from build123d import *

# Parameters (mm, degrees)
SKETCH_R     = 2.8
PAD_DEPTH    = 3
SKETCH001_R  = 1.45
PAD001_DEPTH = 16
POCKET_DEPTH = 2
CHAMFER_SIZE = 0.25


with BuildPart() as part:
    # Sketch → Pad (new body)
    with BuildSketch(Plane.XY):
        Circle(SKETCH_R)
    extrude(amount=PAD_DEPTH)

    # Sketch001 (on Face3 of Pad) → Pad001 (join)
    with BuildSketch(Plane.XY.offset(3)):
        Circle(SKETCH001_R)
    extrude(amount=PAD001_DEPTH)

    # Sketch002 (on Face2 of Pad001) → Pocket (cut)
    with BuildSketch(Plane(origin=(0, 0, 0), x_dir=(1, 0, 0), z_dir=(0, 0, -1))):
        Polygon((1.259542, 0.814588), (-0.075682, 1.49809), (-1.335225, 0.683502), (-1.259542, -0.814588), (0.075682, -1.49809), (1.335225, -0.683502), align=None)
    extrude(amount=-POCKET_DEPTH, mode=Mode.SUBTRACT)

    # Chamfer
    chamfer_edges = [part.edges().sort_by_distance(p)[0] for p in [
        (-2.8, 0, 3),
        (-2.8, 0, 0),
        (1.297384, -0.065543, 0),
        (0.705454, 1.090796, 0),
        (-0.59193, 1.156339, 0),
        (-1.297384, 0.065543, 0),
        (-0.705454, -1.090796, 0),
        (0.59193, -1.156339, 0),
        (-1.45, 0, 19),
    ]]
    chamfer(chamfer_edges, length=CHAMFER_SIZE)


solid = part.part
Read the model definition and answer for the solid it produces. Units are mm, in the model's axes. A direction names the side the tool comes from. Coordinates: 2 decimals unless noted, no trailing zeros. Loops run counter-clockwise (first coordinate to the right, second up) from the corner with the lowest first, then second, coordinate; pieces in that order, holes last.
Q1. Which of the six approach directions +Z, -Z, +X, -X, +Y, -Y give full straight-line access (tool end or side, diameter ignored) to faces 1 (the face through (0, 0, 19)), 2 (the face through (0, -2, 3)), 3 (the face through (0.697, 1.096, 1.113))?
Q2. The part is cut by section C-C on z = 2.25. Write down the section's boundary in (x, y).
Q3. The part is cut by section B-B on z = 6.25. Write down the section's boundary in (x, y).
Q4. Each of these flat-tipped pins is pushed along its axis until it touches: pin 1 Ø1 at (x, y) = (1.5, -1.5) entering from +Z; pin 2 Ø2 at (y, z) = (-0.5, 10.5) entering from +X; pin 3 Ø1 at (x, z) = (0.5, 8.5) entering from +Y. Where does it stop, or does it pass through?
Q5. The part is cut by section A-A on y = 0. Write down the section's boundary in (x, z), and give its area (3 significant figures).
Q6. The mould has two halves that part along X. Classify faces 4 (the face through (2, 0, 0)), 5 (the face through (-1.45, 0.06, 10.76)), 6 (the face through (-0.76, -1.2, 0.13)): +X half, -X half, draft (parallel to the pull), parting line (faces both ways), or undercut.
Q7. Consider probe 1 along Z at (x, y) = (1.6, -0.1); probe 2 along Y at (x, z) = (0.95, 4.25); probe 3 along Z at (x, y) = (-0.15, -1.15). Determine where each line is inside the solid, lowest interval first.
Results below:
1. face 1: +Z, +X, -X, +Y, -Y
1. face 2: +Z
1. face 3: -Z
2. outline: circle Ø5.6 at (0, 0)
3. outline: circle Ø2.9 at (0, 0)
4. pin 1: stops at z = 3
4. pin 2: stops at x = 1.45
4. pin 3: stops at y = 1.45
5. outline: (-2.8, 0.25) - (-2.55, 0) - (-1.55, 0) - (-1.3, 0.25) - (-1.3, 2) - (1.3, 2) - (1.3, 0.25) - (1.55, 0) - (2.55, 0) - (2.8, 0.25) - (2.8, 2.75) - (2.55, 3) - (1.45, 3) - (1.45, 18.75) - (1.2, 19) - (-1.2, 19) - (-1.45, 18.75) - (-1.45, 3) - (-2.55, 3) - (-2.8, 2.75) - close
5. area: 57.7 mm2
6. face 4: draft
6. face 5: parting line
6. face 6: undercut
7. probe 1: z = 0 to 3
7. probe 2: y = -1.1 to 1.1
7. probe 3: z = 2 to 19
